Geometry check sheet. Reference: the model listing, model coordinates, mm. A direction names the side the tool comes from. Give positions to 0.01 mm unless a question says otherwise; leave off trailing zeros. Loops run counter-clockwise (first coordinate to the right, second up) from the corner with the lowest first, then second, coordinate; pieces in that order, holes last. Notation, with made-up numbers: (21.25, 69) -> (73.25, 69) arc R22 cw to (73.25, 89) -> close; hole circle Ø7 at (-19, -4). An arc over 180 degrees is marked (long way). One line per item, written item: value. Start each with the question number.
(1) Sectioned sample at D-D, the plane z = 19.5. Record the cut outline in (x, y), then the cut area to 3 significant figures.
(2) Tool access check on faces 1 (the face through (9.45, 7, 0)), 2 (the face through (15.041, 7.928, 37.135)), 3 (the face through (13.971, 6.886, 38.414)). Record the directions out of +Z, -Z, +X, -X, +Y, -Y that give a thin tool (end or side, any length) a straight path to the whole face; none if there is none.
(3) Gauge pin test, flat ends, axial feed: pin 1 Ø10 at (x, z) = (12, 2) entering from -Y; pin 2 Ø1.2 at (y, z) = (7.5, 19) entering from +X; pin 3 Ø1.8 at (x, z) = (12.45, 41) entering from -Y; pin 4 Ø3 at (x, z) = (11.5, 41) entering from -Y. Record the tip position at first contact, or that the pin passes through.
(4) Scan lines: line 1 along Y through (x, z) = (0, 34); line 2 along Z through (x, y) = (13.25, 7.5); line 3 along X through (y, z) = (8.8, 41). Record each from-to range of solid material in increasing order. Write a range as from..to.
(5) Sectioned sample at A-A, the plane y = 0. Record the cut outline in (x, z), then the cut area to 3 significant figures.
(6) Sectioned sample at C-C, the plane x = -4. Record the cut outline in (y, z).
(7) Draft check along Y on faces 4 (the face through (-6.269, -4.807, 20.115)), 5 (the face through (19, 8, -3)). Enter one of: pulls with the +Y half, pulls with the -Y half, needs draft (parallel to the pull), parting line crosses it, or undercut.
(8) Sectioned sample at B-B, the plane z = 0. Record the cut outline in (x, y), then the cut area to 3 significant figures.
from build123d import *

# Parameters (mm, degrees)
EXTRUDE_1_DEPTH      = 48
EXTRUDE_1_DEPTH_BACK = 7
SKETCH_2_R           = 9.9
SKETCH_2_R_2         = 7.9
CUT_EXTRUDE_1_DEPTH  = 2
SKETCH_4_R           = 1.5
CUT_EXTRUDE_2_DEPTH  = 10
CUT_EXTRUDE_3_DEPTH  = 10


with BuildPart() as part:
    # Эскиз2 → Бобышка-Вытянуть1 (new, two sides: drawn at the far end of the back side and taken through both)
    # profile 1 of 2: a face of its own
    with BuildSketch(Plane.XY.offset(-EXTRUDE_1_DEPTH_BACK)):
        Circle(SKETCH_2_R)
        Circle(SKETCH_2_R_2, mode=Mode.SUBTRACT)
    # profile 2 of 2: a face of its own
    with BuildSketch(Plane.XY.offset(-EXTRUDE_1_DEPTH_BACK)):
        with BuildLine():
            Line((19, 9.9), (0, 9.9))
            ThreePointArc((0, 9.9), (4.449719092, 8.843641784), (7.949842766, 5.9))
            Line((7.949842766, 5.9), (19, 5.9))
            Line((19, 5.9), (19, 9.9))
        make_face()
    extrude(amount=EXTRUDE_1_DEPTH + EXTRUDE_1_DEPTH_BACK)

    # Эскиз3 → Вырез-Вытянуть1 (cut)
    with BuildSketch(Plane.XZ.offset(-5.9)):
        Polygon((15.449842766, -1.732050808), (15.449842766, 1.732050808), (12.449842766, 3.464101615), (9.449842766, 1.732050808), (9.449842766, -1.732050808), (12.449842766, -3.464101615), align=None)
        Polygon((12.449842766, 44.464101615), (15.449842766, 42.732050808), (15.449842766, 39.267949192), (12.449842766, 37.535898385), (9.449842766, 39.267949192), (9.449842766, 42.732050808), align=None)
    extrude(amount=-CUT_EXTRUDE_1_DEPTH, mode=Mode.SUBTRACT)

    # Эскиз4 → Вырез-Вытянуть2 (cut)
    with BuildSketch(Plane(origin=(0, 9.9, 0), x_dir=(1, 0, 0), z_dir=(0, 1, 0))):
        with Locations(Location((12.449842766, 0, 0), (0, 0, 270))):
            Circle(SKETCH_4_R)
        with Locations(Location((12.449842766, -41, 0), (0, 0, 270))):
            Circle(SKETCH_4_R)
    extrude(amount=-CUT_EXTRUDE_2_DEPTH, mode=Mode.SUBTRACT)

    # Эскиз5 → Вырез-Вытянуть3 (cut)
    with BuildSketch(Plane(origin=(0, 9.9, 0), x_dir=(1, 0, 0), z_dir=(0, 1, 0))):
        Polygon((19, -1.578851944), (11.190820694, -6.087483718), (11.190820694, -34.912516282), (19, -39.421148056), align=None)
    extrude(amount=-CUT_EXTRUDE_3_DEPTH, mode=Mode.SUBTRACT)


solid = part.part
Calculated:
1. outline: (0, 9.9) arc R9.9 ccw (long way) to (7.95, 5.9) -> (11.19, 5.9) -> (11.19, 9.9) -> close; hole circle Ø15.8 at (0, 0)
1. area: 134 mm2
2. face 1: none
2. face 2: +X, +Y, -Y
2. face 3: -Y
3. pin 1: stops at y = -7
3. pin 2: stops at x = 11.19
3. pin 3: passes through
3. pin 4: stops at y = 7.9
4. line 1: y = -9.9..-7.9, 7.9..9.9
4. line 2: z = -7..-3, 3..4.9, 36.1..38, 44..48
4. line 3: x = -4.54..10.95, 13.95..19
5. outline: (-9.9, -7) -> (-7.9, -7) -> (-7.9, 48) -> (-9.9, 48) -> close; (7.9, -7) -> (9.9, -7) -> (9.9, 48) -> (7.9, 48) -> close
5. area: 220 mm2
6. outline: (-9.06, -7) -> (-6.81, -7) -> (-6.81, 48) -> (-9.06, 48) -> close; (6.81, -7) -> (9.06, -7) -> (9.06, 48) -> (6.81, 48) -> close
7. face 4: undercut
7. face 5: needs draft
8. outline: (0, 9.9) arc R9.9 ccw (long way) to (7.95, 5.9) -> (9.45, 5.9) -> (9.45, 7.9) -> (10.95, 7.9) -> (10.95, 9.9) -> close; (13.95, 7.9) -> (15.45, 7.9) -> (15.45, 5.9) -> (19, 5.9) -> (19, 9.9) -> (13.95, 9.9) -> close; hole circle Ø15.8 at (0, 0)
8. area: 148 mm2
